Geometry check sheet. Reference: the model listing, model coordinates, mm. Face numbers are marked on the shaded views. A direction names the side the tool comes from. Round coordinates to 2 decimals unless told otherwise and drop trailing zeros. Order: outer loops, then holes, each group sorted by start corner. A loop starts at its lowest first (then second) coordinate and runs counter-clockwise, first axis right, second up. Notation, with made-up numbers: (68.25, -31) -> (93.25, -31) arc R15 ccw to (93.25, -11) -> close; hole circle Ø2 at (-19.5, 44.5). An arc over 180 degrees is marked (long way). Use a Markdown table: item, result. Add a question column.
Item 1: Sectioned sample at A-A, the plane x = -8.96. Record the cut outline in (y, z) (3 decimals), and give its area (3 significant figures).
Item 2: Sectioned sample at B-B, the plane y = 1.5. Record the cut outline in (x, z).
Item 3: Gauge pin test, flat ends, axial feed: pin 1 Ø2 at (y, z) = (37.5, 8.5) entering from +X; pin 2 Ø2 at (x, z) = (32.5, 6.5) entering from +Y; pin 3 Ø0.6 at (x, y) = (0.5, 37) entering from +Z. Record the tip position at first contact, or that the pin passes through.
Item 4: Mould release check, pull along X, two halves, no side actions. Record for the marked faces 1, 2 and 3: pulls with the +X half, pulls with the -X half, needs draft (parallel to the pull), parting line crosses it, or undercut.
Item 5: Set-up check for the marked faces 4 and 5: record each of +Z, -Z, +X, -X, +Y, -Y from which the full face is reachable in a straight line by a thin tool's end or side.
Item 6: Material ranges on probe 1 along X at (y, z) = (-6, 5.5); probe 2 along Y at (x, z) = (-18, 8.5); probe 3 along Y at (x, z) = (31, 8), recorded low to high. Write a range as [from, to].
Item 7: Sectioned sample at C-C, the plane z = 11.75. Record the cut outline in (x, y), and give its area (3 significant figures).
Item 8: Sectioned sample at D-D, the plane x = 18.94. Record the cut outline in (y, z).
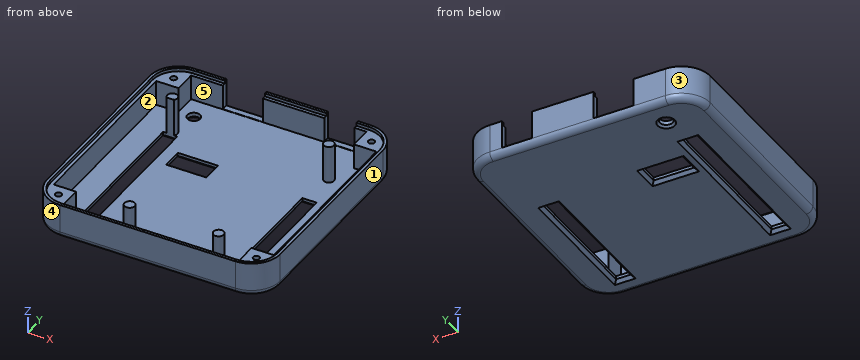
from build123d import *

# Parameters (mm, degrees)
F1_DEPTH  = 2
F2_R      = 1.6
F3_DEPTH  = 11.8
F5_DEPTH  = 8.9
F7_DEPTH  = 1
F8_W      = 12.6
F8_H      = 2
F8_W_2    = 9.5
F9_DEPTH  = 8.8
F10_W     = 4.5
F10_H     = 49.5
F10_H_2   = 40.5
F11_DEPTH = 10
F12_DEPTH = 15
F14_DEPTH = 7.9
F15_R     = 1
F16_DEPTH = 7
F17_W     = 12.6
F17_H     = 6.5
F18_DEPTH = 4
F19_SIZE  = 1
F20_R     = 2
F21_DEPTH = 4
F22_R     = 2
F23_SIZE  = 0.7


with BuildPart() as f1:
    # F0 (on Top) → F1 (new body)
    with BuildSketch(Plane.XY):
        with BuildLine():
            Line((27.5, 38.5), (-27.5, 38.5))
            ThreePointArc((-27.5, 38.5), (-33.863961, 35.863961), (-36.5, 29.5))
            Line((-36.5, 29.5), (-36.5, -27.5))
            ThreePointArc((-36.5, -27.5), (-33.863961, -33.863961), (-27.5, -36.5))
            Line((-27.5, -36.5), (27.5, -36.5))
            ThreePointArc((27.5, -36.5), (33.863961, -33.863961), (36.5, -27.5))
            Line((36.5, -27.5), (36.5, 29.5))
            ThreePointArc((36.5, 29.5), (33.863961, 35.863961), (27.5, 38.5))
        make_face()
    extrude(amount=F1_DEPTH)

    # F2 (on face) → F3 (join)
    with BuildSketch(Plane.XY.offset(2)):
        with Locations((-24.16, 20.2)):
            Circle(F2_R)
        with Locations((24.14, 21.5)):
            Circle(F2_R)
        with Locations((18.94, -30.6)):
            Circle(F2_R)
        with Locations((-8.96, -30.6)):
            Circle(F2_R)
    extrude(amount=F3_DEPTH)

    # F4 (on face) → F5 (join)
    with BuildSketch(Plane.XY.offset(2)):
        with BuildLine():
            Line((27.5, 38.5), (-27.5, 38.5))
            ThreePointArc((-27.5, 38.5), (-33.863961, 35.863961), (-36.5, 29.5))
            Line((-36.5, 29.5), (-36.5, -27.5))
            ThreePointArc((-36.5, -27.5), (-33.863961, -33.863961), (-27.5, -36.5))
            Line((-27.5, -36.5), (27.5, -36.5))
            ThreePointArc((27.5, -36.5), (33.863961, -33.863961), (36.5, -27.5))
            Line((36.5, -27.5), (36.5, 29.5))
            ThreePointArc((36.5, 29.5), (33.863961, 35.863961), (27.5, 38.5))
        make_face()
        with BuildLine():
            ThreePointArc((-34.5, 29.5), (-32.449747, 34.449747), (-27.5, 36.5))
            Line((-27.5, 36.5), (27.5, 36.5))
            ThreePointArc((27.5, 36.5), (32.449747, 34.449747), (34.5, 29.5))
            Line((34.5, 29.5), (34.5, -27.5))
            ThreePointArc((34.5, -27.5), (32.449747, -32.449747), (27.5, -34.5))
            Line((27.5, -34.5), (-27.5, -34.5))
            ThreePointArc((-27.5, -34.5), (-32.449747, -32.449747), (-34.5, -27.5))
            Line((-34.5, -27.5), (-34.5, 29.5))
        make_face(mode=Mode.SUBTRACT)
    extrude(amount=F5_DEPTH)

    # F6 (on face) → F7 (cut)
    with BuildSketch(Plane.XY.offset(10.9)):
        with BuildLine():
            Line((27.5, 37.6), (-27.5, 37.6))
            ThreePointArc((-27.5, 37.6), (-33.227565, 35.227565), (-35.6, 29.5))
            Line((-35.6, 29.5), (-35.6, -27.5))
            ThreePointArc((-35.6, -27.5), (-33.227565, -33.227565), (-27.5, -35.6))
            Line((-27.5, -35.6), (27.5, -35.6))
            ThreePointArc((27.5, -35.6), (33.227565, -33.227565), (35.6, -27.5))
            Line((35.6, -27.5), (35.6, 29.5))
            ThreePointArc((35.6, 29.5), (33.227565, 35.227565), (27.5, 37.6))
        make_face()
        with BuildLine():
            ThreePointArc((-34.5, 29.5), (-32.449747, 34.449747), (-27.5, 36.5))
            Line((-27.5, 36.5), (27.5, 36.5))
            ThreePointArc((27.5, 36.5), (32.449747, 34.449747), (34.5, 29.5))
            Line((34.5, 29.5), (34.5, -27.5))
            ThreePointArc((34.5, -27.5), (32.449747, -32.449747), (27.5, -34.5))
            Line((27.5, -34.5), (-27.5, -34.5))
            ThreePointArc((-27.5, -34.5), (-32.449747, -32.449747), (-34.5, -27.5))
            Line((-34.5, -27.5), (-34.5, 29.5))
        make_face(mode=Mode.SUBTRACT)
    extrude(amount=-F7_DEPTH, mode=Mode.SUBTRACT)

    # F8 (on face) → F9 (cut)
    with BuildSketch(Plane.XY.offset(10.9)):
        with Locations((-11.26, 37.5)):
            Rectangle(F8_W, F8_H)
        with Locations((18.99, 37.5)):
            Rectangle(F8_W_2, F8_H)
    extrude(amount=-F9_DEPTH, mode=Mode.SUBTRACT)

    # F10 (on face) → F11 (cut)
    with BuildSketch(Plane.XY.offset(2)):
        with Locations((-24.21, -5.65)):
            Rectangle(F10_W, F10_H)
        with Locations((24.49, -10.15)):
            Rectangle(F10_W, F10_H_2)
    extrude(amount=-F11_DEPTH, mode=Mode.SUBTRACT)

    # F10 (on face) → F12 (cut)
    with BuildSketch(Plane.XY.offset(2)):
        with Locations((-24.21, -5.65)):
            Rectangle(F10_W, F10_H)
        with Locations((24.49, -10.15)):
            Rectangle(F10_W, F10_H_2)
    extrude(amount=F12_DEPTH, mode=Mode.SUBTRACT)

    # F13 (on face) → F14 (join)
    with BuildSketch(Plane.XY.offset(2)):
        with BuildLine():
            Line((-27.5, 29.5), (-27.5, 36.5))
            ThreePointArc((-27.5, 36.5), (-32.449747, 34.449747), (-34.5, 29.5))
            Line((-34.5, 29.5), (-27.5, 29.5))
        make_face()
        with BuildLine():
            Line((27.5, 29.5), (34.5, 29.5))
            ThreePointArc((34.5, 29.5), (32.449747, 34.449747), (27.5, 36.5))
            Line((27.5, 36.5), (27.5, 29.5))
        make_face()
        with BuildLine():
            Line((27.5, -27.5), (27.5, -34.5))
            ThreePointArc((27.5, -34.5), (32.449747, -32.449747), (34.5, -27.5))
            Line((34.5, -27.5), (27.5, -27.5))
        make_face()
        with BuildLine():
            Line((-27.5, -27.5), (-34.5, -27.5))
            ThreePointArc((-34.5, -27.5), (-32.449747, -32.449747), (-27.5, -34.5))
            Line((-27.5, -34.5), (-27.5, -27.5))
        make_face()
    extrude(amount=F14_DEPTH)

    # F15 (on face) → F16 (cut)
    with BuildSketch(Plane.XY.offset(9.9)):
        with Locations((-31, 33)):
            Circle(F15_R)
        with Locations((31, 33)):
            Circle(F15_R)
        with Locations((31, -31)):
            Circle(F15_R)
        with Locations((-31, -31)):
            Circle(F15_R)
    extrude(amount=-F16_DEPTH, mode=Mode.SUBTRACT)

    # F17 (on face) → F18 (cut)
    with BuildSketch(Plane.XY.offset(2)):
        with Locations((-11.76, 9.075)):
            Rectangle(F17_W, F17_H)
    extrude(amount=-F18_DEPTH, mode=Mode.SUBTRACT)

    # F19
    f19_edges = [f1.edges().sort_by_distance(p)[0] for p in [
        (-26.46, -5.65, 0),
        (-24.21, 19.1, 0),
        (-21.96, -5.65, 0),
        (-24.21, -30.4, 0),
        (-11.76, 5.825, 0),
        (-18.06, 9.075, 0),
        (-11.76, 12.325, 0),
        (-5.46, 9.075, 0),
        (22.24, -10.15, 0),
        (26.74, -10.15, 0),
        (24.49, 10.1, 0),
        (24.49, -30.4, 0),
    ]]
    chamfer(f19_edges, length=F19_SIZE)

    # F20 (on face) → F21 (cut)
    with BuildSketch(Plane.XY.offset(2)):
        with Locations((-22.7, 29.5)):
            Circle(F20_R)
    extrude(amount=-F21_DEPTH, mode=Mode.SUBTRACT)

    # F22
    f22_edges = [f1.edges().sort_by_distance(p)[0] for p in [
        (0, 38.5, 0),
    ]]
    fillet(f22_edges, radius=F22_R)

    # F23
    f23_edges = [f1.edges().sort_by_distance(p)[0] for p in [
        (-24.7, 29.5, 0),
    ]]
    chamfer(f23_edges, length=F23_SIZE)


solid = f1.part
Found:
| question | item | result |
|---|---|---|
| 1 | outline | (-36.5, 2) arc R2 ccw to (-34.5, 0) -> (4.825, 0) -> (5.825, 1) -> (5.825, 2) -> (-29, 2) -> (-29, 13.8) -> (-32.2, 13.8) -> (-32.2, 2) -> (-34.5, 2) -> (-34.5, 9.9) -> (-35.6, 9.9) -> (-35.6, 10.9) -> (-36.5, 10.9) -> close; (12.325, 1) -> (13.325, 0) -> (36.5, 0) arc R2 ccw to (38.5, 2) -> (38.5, 2.1) -> (36.5, 2.1) -> (36.5, 2) -> (12.325, 2) -> close |
| 1 | area | 189 mm2 |
| 2 | outline | (-36.5, 2) arc R2 ccw to (-34.5, 0) -> (-27.46, 0) -> (-26.46, 1) -> (-26.46, 2) -> (-34.5, 2) -> (-34.5, 9.9) -> (-35.6, 9.9) -> (-35.6, 10.9) -> (-36.5, 10.9) -> close; (-21.96, 1) -> (-20.96, 0) -> (21.24, 0) -> (22.24, 1) -> (22.24, 2) -> (-21.96, 2) -> close; (26.74, 1) -> (27.74, 0) -> (34.5, 0) arc R2 ccw to (36.5, 2) -> (36.5, 10.9) -> (35.6, 10.9) -> (35.6, 9.9) -> (34.5, 9.9) -> (34.5, 2) -> (26.74, 2) -> close |
| 3 | pin 1 | stops at x = 33.16 |
| 3 | pin 2 | stops at y = 37.56 |
| 3 | pin 3 | stops at z = 9.9 |
| 4 | face 1 | pulls with the +X half |
| 4 | face 2 | undercut |
| 4 | face 3 | pulls with the -X half |
| 5 | face 4 | +Z, -Z, -X, -Y |
| 5 | face 5 | +Z |
| 6 | probe 1 | x = [-36.5, -34.5], [34.5, 36.5] |
| 6 | probe 2 | y = [-36.5, -34.5], [36.5, 38.5] |
| 6 | probe 3 | y = [-35.79, -32], [-30, -27.5], [29.5, 32], [34, 37.79] |
| 7 | outline | (-25.32, 19.1) -> (-23, 19.1) arc R1.6 ccw (long way) to start; circle Ø3.2 at (-8.96, -30.6); circle Ø3.2 at (18.94, -30.6); circle Ø3.2 at (24.14, 21.5) |
| 7 | area | 31.4 mm2 |
| 8 | outline | (-36.5, 2) arc R2 ccw to (-34.5, 0) -> (36.5, 0) arc R2 ccw to (38.5, 2) -> (38.5, 2.1) -> (36.5, 2.1) -> (36.5, 2) -> (-29, 2) -> (-29, 13.8) -> (-32.2, 13.8) -> (-32.2, 2) -> (-34.5, 2) -> (-34.5, 9.9) -> (-35.6, 9.9) -> (-35.6, 10.9) -> (-36.5, 10.9) -> close |
